Verification items for the finished model (mm, model axes). A direction names the side the tool comes from. Round coordinates to 2 decimals unless told otherwise and drop trailing zeros. Order: outer loops, then holes, each group sorted by start corner. A loop starts at its lowest first (then second) coordinate and runs counter-clockwise, first axis right, second up. Notation, with made-up numbers: M -5.5,28 L 4.5,28 A10 ccw 4.5,33 Z; hole C 23,67 d8. An arc over 180 degrees is marked long. Use CSV: the item, a comma, the result in double quotes. Start each with the question number.
Q1. Sectioned sample at A-A (x = -37.25). Enter the section's corners in (y, z), and give its area (3 significant figures).
Q2. Sectioned sample at C-C (x = 9). Enter the section's corners in (y, z), and give its area (3 significant figures).
Q3. Scan lines: line 1 (Y direction, x = -37.25, z = -1.15); line 2 (X direction, y = -13.25, z = -3); line 3 (Z direction, x = -11, y = -6.75). Record each from-to range of solid material in increasing order.
Q4. Gauge pin test, flat ends, axial feed: pin 1 Ø4.5 at (x, y) = (-37.25, -7.5) entering from +Z; pin 2 Ø4.5 at (y, z) = (-4.5, -4.5) entering from -X; pin 3 Ø1 at (y, z) = (-5.5, -3.5) entering from -X; pin 4 Ø3 at (x, z) = (-19.5, -5) entering from -Y. Record the tip position at first contact, or that the pin passes through.
Q5. Set-up check for faces 1 (the face through (-0.25, -7, -3)), 2 (the face through (41, -7, -6.5)), 3 (the face through (-23, -7, -2)), 4 (the face through (40.25, -7, -3)), 5 (the face through (-38.877, -8.747, -0.993)): record each of +Z, -Z, +X, -X, +Y, -Y from which the full face is reachable in a straight line by a thin tool's end or side.
Q6. Mould release check, pull along X, two halves, no side actions. Record for faces 6 (the face through (42.25, -7, -3)), 7 (the face through (20, -7, -2)), 8 (the face through (1, -7, 0)): +X half, -X half, draft (parallel to the pull), parting line (faces both ways), or undercut.
```python
from build123d import *

# Parameters (mm, degrees)
F1_DEPTH = 15
F2_R     = 2.05
F3_DEPTH = 25
F4_R     = 0.49999


# Not quite as in the source:
# - a fillet or chamfer is up to 0.001 mm smaller than in the source, because OpenCascade refuses the exact size


with BuildPart() as f1:
    # F0 (on Front) → F1 (new body)
    with BuildSketch(Plane.XZ):
        Polygon((-0.25, -2), (-2.25, -2), (-2.25, -8.6), (-0.25, -8.6), (-0.25, -6.6), (-1.25, -6.6), (-1.25, -4.4), (-0.25, -4.4), align=None)
        Polygon((42.25, 0), (-42.25, 0), (-42.25, -2), (-2.25, -2), (-0.25, -2), (40.25, -2), (42.25, -2), align=None)
        Polygon((42.25, -6.5), (42.25, -2), (40.25, -2), (40.25, -4.5), (39.75, -4.5), (39.75, -6.5), align=None)
    extrude(amount=F1_DEPTH)

    # F2 (on face) → F3 (cut)
    with BuildSketch(Plane.XY):
        with Locations((-37.25, -7.5)):
            Circle(F2_R)
    extrude(amount=-F3_DEPTH, mode=Mode.SUBTRACT)

    # F4 (radius 0.5 in the source; OpenCascade refuses exactly that, so slightly less here)
    f4_edges = [f1.edges().sort_by_distance(p)[0] for p in [
        (-1.25, -7.5, -6.6),
        (-0.25, -7.5, -8.6),
        (39.75, -7.5, -6.5),
        (39.75, -7.5, -4.5),
        (-39.3, -7.5, 0),
        (42.25, -7.5, 0),
        (42.25, -7.5, -6.5),
        (-42.25, -7.5, 0),
        (-42.25, -7.5, -2),
        (-2.25, -7.5, -2),
        (-0.25, -7.5, -2),
        (40.25, -7.5, -2),
        (-2.25, -7.5, -8.6),
        (-39.3, -7.5, -2),
        (-0.25, -7.5, -4.4),
        (-1.25, -7.5, -4.4),
        (-0.25, -7.5, -6.6),
    ]]
    fillet(f4_edges, radius=F4_R)


solid = f1.part
```
Verdict:
1,outline,"M -15,-2 L -10.05,-2 A0.5 ccw -9.55,-1.5 L -9.55,-0.5 A0.5 ccw -10.05,0 L -15,0 Z; M -5.45,-1.5 A0.5 ccw -4.95,-2 L 0,-2 L 0,0 L -4.95,0 A0.5 ccw -5.45,-0.5 Z"
1,area,"21.6 mm²"
2,outline,"M -15,-2 L 0,-2 L 0,0 L -15,0 Z"
2,area,"30.0 mm²"
3,line 1,"y = -15 to -9.55, -5.45 to 0"
3,line 2,"x = -2.25 to -0.25, 40.25 to 42.25"
3,line 3,"z = -2 to 0"
4,pin 1,"stops at z = -0.1"
4,pin 2,"stops at x = -2.32"
4,pin 3,"stops at x = -2.25"
4,pin 4,"passes through"
5,face 1,"-Z, +Y, -Y"
5,face 2,"-Z, +X, +Y, -Y"
5,face 3,"-Z, -X, +Y, -Y"
5,face 4,"+Y, -Y"
5,face 5,"+Z, -Z"
6,face 6,"+X half"
6,face 7,"undercut"
6,face 8,"draft"
